Solid Edge part; units mm, degrees
sketch "Sketch1" plane through (0, 0, 0) normal (0, -1, 0) x (1, 0, 0)
  circle A0 centre (80.5127, 55.3877) radius 22.5
extrude "ExtrudedProtrusion_1" add sketch "Sketch1" against normal blind 10
sketch "Sketch2" plane through (63.9305, 0, 41.9251) normal (0, -1, 0) x (1, 0, 0)
  line L0 (18.5822, 5.9759) -> (18.5822, 0.9759)
  arc A0 (18.5822, 0.9759) -> (14.5822, 0.9759) centre (16.5822, 0.9759) cw
  line L1 (14.5822, 0.9759) -> (14.5822, 5.9759)
  arc A1 (14.5822, 5.9759) -> (9.5822, 10.9759) centre (9.5822, 5.9759) ccw
  line L2 (9.5822, 10.9759) -> (4.5822, 10.9759)
  arc A2 (4.5822, 10.9759) -> (4.5822, 14.9759) centre (4.5822, 12.9759) cw
  line L3 (4.5822, 14.9759) -> (9.5822, 14.9759)
  arc A3 (9.5822, 14.9759) -> (12.5822, 17.9759) centre (9.5822, 17.9759) ccw
  arc A4 (12.5822, 17.9759) -> (20.5822, 17.9759) centre (16.5822, 13.4626) cw
  arc A5 (23.5822, 14.9759) -> (20.5822, 17.9759) centre (23.5822, 17.9759) cw
  line L4 (28.5822, 14.9759) -> (23.5822, 14.9759)
  arc A6 (28.5822, 10.9759) -> (28.5822, 14.9759) centre (28.5822, 12.9759) ccw
  line L5 (23.5822, 10.9759) -> (28.5822, 10.9759)
  arc A7 (18.5822, 5.9759) -> (23.5822, 10.9759) centre (23.5822, 5.9759) cw
  dimension "D1" = 18.5822
  dimension "D2" = 14.5822
  dimension "D3" = 23.5822
  dimension "D4" = 9.5822
  dimension "D5" = 4.5822
  dimension "D6" = 28.5822
extrude "Cutout1" cut sketch "Sketch2" against normal blind 5
sketch "Sketch3" plane through (80.5127, 10, 55.3877) normal (0, 1, 0) x (0, 0, -1)
  circle A0 centre (0, 0) radius 3
extrude "ExtrudedCutout_5" cut sketch "Sketch3" against normal blind 3
sketch "Sketch4" plane through (80.5127, 7, 55.3877) normal (0, 1, 0) x (-1, 0, 0)
  circle A0 centre (0, 0) radius 1.05
extrude "Cutout2" cut sketch "Sketch4" against normal up to next
sketch "Sketch5" plane through (80.5127, 5, 51.1598) normal (0, -1, 0) x (1, 0, 0)
  circle A0 centre (0, 4.2279) radius 3.55
extrude "ExtrudedCutout_7" cut sketch "Sketch5" against normal blind 0.5
chamfer "Chamfer_2" distance 1.9 distance2 0.5 1 edges at (80.5127, 7, 58.3877) measured on face at (78.5727, 7, 53.3277)
Could you check a few things on this model? Use its own coordinates, in mm. A direction names the side the tool comes from. Coordinates: 2 decimals unless noted, no trailing zeros. Write each loop counter-clockwise with the first axis right and the second up, starting at its lowest first coordinate (ties: lowest second). Pieces come first, ordered by that corner, then holes. Notation, with made-up numbers: (78, 16.25) - (82, 16.25) arc R8 ccw to (82, 26.25) - close; hole circle Ø2 at (41.25, -29). An arc over 180 degrees is marked (long way). Write item = value, one per line.
1) Suppose I cut it at D-D on x = 63.5. Please give me the cut outline in (y, z).
Result set:
outline = (0, 40.66) - (10, 40.66) - (10, 70.11) - (0, 70.11) - close
2) Suppose I cut it at B-B on x = 86. Please give me the cut outline in (y, z), plus the area to 3 significant figures.
Result set:
outline = (0, 33.57) - (10, 33.57) - (10, 77.21) - (0, 77.21) - (0, 57.31) - (5, 57.31) - (5, 52.67) - (0, 52.67) - close
area = 413 mm2
3) We'd pull the mould along X, two halves only. Please class faces 1 (the flat face through (90, 2, 52.901)), 2 (the cylindrical face through (81.287, 6.26, 56.097)), 3 (the flat face through (76, 10, 56)): +X half, -X half, draft (parallel to the pull), parting line (faces both ways), or undercut.
Result set:
face_1 = undercut
face_2 = undercut
face_3 = draft
4) Suppose I cut it at C-C on z = 66.5. Please give me the cut outline in (x, y), plus the area to 3 significant figures.
Result set:
outline = (60.95, 0) - (100.08, 0) - (100.08, 10) - (60.95, 10) - close
area = 391 mm2
5) Please list where these lines run through material, in increasing order: line 1 (Z direction, x = 80.5, y = 5.25); line 2 (Z direction, x = 83, y = 3.25); line 3 (X direction, y = 1.5, z = 47). Write a range as [from, to].
Result set:
line_1 = [32.89, 51.84], [58.94, 77.89]
line_2 = [33.03, 50.05], [60.88, 77.75]
line_3 = [59.63, 78.51], [82.51, 101.39]
6) Will these pins go through, and if not, where does the flat tip stop? pin 1 Ø6 at (x, y) = (70, 2.5) entering from -Z; pin 2 Ø5 at (x, y) = (96.5, 6) entering from +Z; pin 3 Ø5.5 at (x, y) = (70.5, 3.5) entering from +Z.
Result set:
pin_1 = 34.18
pin_2 = 73.4
pin_3 = 76.68
7) Suppose I cut it at A-A on y = 3.5. Please give me the cut outline in (x, z), plus the area to 3 significant figures.
Result set:
outline = circle Ø45 at (80.51, 55.39); hole (68.51, 52.9) - (73.51, 52.9) arc R5 cw to (78.51, 47.9) - (78.51, 42.9) arc R2 ccw to (82.51, 42.9) - (82.51, 47.9) arc R5 cw to (87.51, 52.9) - (92.51, 52.9) arc R2 ccw to (92.51, 56.9) - (87.51, 56.9) arc R3 cw to (84.51, 59.9) arc R6.03 ccw to (76.51, 59.9) arc R3 cw to (73.51, 56.9) - (68.51, 56.9) arc R2 ccw to start
area = 1,390 mm2
8) For faces 4 (the flat face through (71, 2, 56.901)), 5 (the flat face through (76, 0, 51)), 6 (the cylindrical face through (83.174, 8.768, 54.003)), which set-ups out of +Z, -Z, +X, -X, +Y, -Y let a thin tool reach every point of the face, with its end or its side?
Result set:
face_4 = -Y
face_5 = +Z, -Z, +X, -X, -Y
face_6 = +Y
